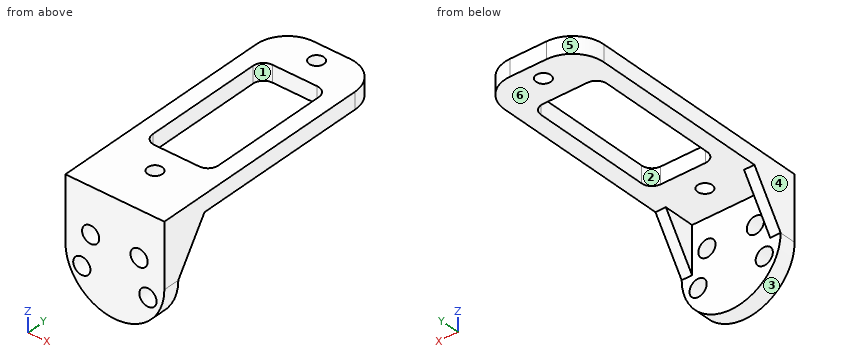
from build123d import *

# Parameters (mm, degrees)
SKETCH1_R               = 1.4
BOSS_EXTRUDE1_DEPTH     = 3.2
BOSS_EXTRUDE3_DEPTH     = 3.2
BOSS_EXTRUDE4_DEPTH     = 2
LPATTERN1_COUNT         = 2
LPATTERN1_PITCH         = 17
CUT_EXTRUDE1_DEPTH      = 54.530365215
CUT_EXTRUDE4_DEPTH      = 54.530365215
CUT_EXTRUDE4_DEPTH_BACK = 54.530365215
SKETCH8_R               = 1.65


with BuildPart() as part:
    # Sketch1 → Boss-Extrude1 (new body)
    with BuildSketch(Plane.XY):
        with BuildLine():
            Line((0, 0), (19, 0))
            Line((19, 0), (19, 40.5))
            ThreePointArc((19, 40.5), (17.242640687, 44.742640687), (13, 46.5))
            Line((13, 46.5), (6, 46.5))
            ThreePointArc((6, 46.5), (1.757359313, 44.742640687), (0, 40.5))
            Line((0, 40.5), (0, 0))
        make_face()
        with Locations((9.5, 6)):
            Circle(SKETCH1_R, mode=Mode.SUBTRACT)
        with Locations((9.5, 43)):
            Circle(SKETCH1_R, mode=Mode.SUBTRACT)
    extrude(amount=BOSS_EXTRUDE1_DEPTH)

    # Sketch2 → Boss-Extrude3 (add)
    with BuildSketch(Plane(origin=(0, 0, 0), x_dir=(1, 0, 0), z_dir=(0, 1, 0))):
        with BuildLine():
            Line((0, 9), (0, -3.2))
            Line((0, -3.2), (19, -3.2))
            Line((19, -3.2), (19, 9))
            ThreePointArc((19, 9), (9.5, 18.5), (0, 9))
        make_face()
    extrude(amount=-BOSS_EXTRUDE3_DEPTH)

    # Sketch3 → Boss-Extrude4 (add)
    with BuildSketch(Plane(origin=(0, 0, 0), x_dir=(0, 0, -1), z_dir=(1, 0, 0))):
        Polygon((0, 0), (9, 0), (0, 6), align=None)
    boss_extrude4 = extrude(amount=BOSS_EXTRUDE4_DEPTH)

    # LPattern1: Boss-Extrude4 ×2
    with Locations(*[(i * LPATTERN1_PITCH, 0, 0) for i in range(1, LPATTERN1_COUNT)]):
        add(boss_extrude4)

    # Sketch4 → Cut-Extrude1 (cut, through all)
    with BuildSketch(Plane.XY):
        with BuildLine():
            Line((5.2, 38), (13.8, 38))
            ThreePointArc((13.8, 38), (15.214213562, 37.414213562), (15.8, 36))
            Line((15.8, 36), (15.8, 13))
            ThreePointArc((15.8, 13), (15.214213562, 11.585786438), (13.8, 11))
            Line((13.8, 11), (5.2, 11))
            ThreePointArc((5.2, 11), (3.785786438, 11.585786438), (3.2, 13))
            Line((3.2, 13), (3.2, 36))
            ThreePointArc((3.2, 36), (3.785786438, 37.414213562), (5.2, 38))
        make_face()
    extrude(amount=CUT_EXTRUDE1_DEPTH, mode=Mode.SUBTRACT)

    # Sketch8 → Cut-Extrude4 (cut, two sides: drawn at the far end of the back side and taken through both)
    with BuildSketch(Plane(origin=(0, 0, 0), x_dir=(1, 0, 0), z_dir=(0, 1, 0)).offset(-CUT_EXTRUDE4_DEPTH_BACK)):
        with Locations(Location((3.15, 11.8, 0), (0, 0, 270))):
            Circle(SKETCH8_R)
        with Locations(Location((14.14852263, 5.45, 0), (0, 0, 270))):
            Circle(SKETCH8_R)
        with Locations(Location((4.85147737, 5.45, 0), (0, 0, 270))):
            Circle(SKETCH8_R)
        with Locations(Location((15.85, 11.8, 0), (0, 0, 270))):
            Circle(SKETCH8_R)
    extrude(amount=CUT_EXTRUDE4_DEPTH + CUT_EXTRUDE4_DEPTH_BACK, mode=Mode.SUBTRACT)


solid = part.part
Source: CAD feature listing. Evaluate the final solid. Frame: model axes, mm. Face numbers are marked on the shaded views. A direction names the side the tool comes from. Round coordinates to 2 decimals unless told otherwise and drop trailing zeros. Loops run counter-clockwise (first coordinate to the right, second up) from the corner with the lowest first, then second, coordinate; pieces in that order, holes last. Notation, with made-up numbers: (38.5, -29.5) -> (64.5, -29.5) arc R17 cw to (64.5, -20.5) -> close; hole circle Ø6 at (10, 20). An arc over 180 degrees is marked (long way). Answer as a JSON object with one key per item and string values. Group by question number.
Q1. Section query A-A (x = 9.5). Output: boundary loops of the cut face in (y, z), plus the area to 3 significant figures.
Q2. Mould query, pull axis X, two halves, no side actions, for the marked faces 1, 2, 3 and 4. Classes: pulls with the +X half, pulls with the -X half, needs draft (parallel to the pull), parting line crosses it, or undercut.
Q3. Contact query for flat-ended pins moving along their axis: P1, Ø6, axis at x = 7.5, z = -11, coming from the +Y side; P2, Ø3, axis at x = 9.5, y = 6, coming from the -Z side. Output: stop coordinate, or through.
Q4. Section query D-D (y = 9). Output: boundary loops of the cut face in (x, z).
Q5. Section query C-C (z = -5.45). Output: boundary loops of the cut face in (x, y), plus the area to 3 significant figures.
Q6. Section query B-B (y = 15). Output: boundary loops of the cut face in (x, z).
Q7. Ray query, line 1 (Y direction, x = 9.5, z = 0.5); line 2 (X direction, y = -2.4, z = -11.8); line 3 (X direction, y = 2, z = -0.25). Return the intervals inside material, ascending. Write a range as from..to.
Q8. Access query for the marked faces 5 and 6. Directions: +Z, -Z, +X, -X, +Y, -Y. A direction counts if a zero-diameter tool reaches every point of the face in a straight line with its end or side. Return the directions, or none.
Completed:
{
 "1": {"outline": "(-3.2, -18.5) -> (0, -18.5) -> (0, 0) -> (4.6, 0) -> (4.6, 3.2) -> (-3.2, 3.2) -> close; (7.4, 0) -> (11, 0) -> (11, 3.2) -> (7.4, 3.2) -> close; (38, 0) -> (41.6, 0) -> (41.6, 3.2) -> (38, 3.2) -> close; (44.4, 0) -> (46.5, 0) -> (46.5, 3.2) -> (44.4, 3.2) -> close", "area": "114 mm²"},
 "2": {"face 1": "undercut", "face 2": "undercut", "face 3": "parting line crosses it", "face 4": "pulls with the -X half"},
 "3": {"P1": "y = 0", "P2": "z = 0"},
 "4": {"outline": "(0, 0) -> (19, 0) -> (19, 3.2) -> (0, 3.2) -> close"},
 "5": {"outline": "(0, -3.2) -> (3.2, -3.2) -> (3.2, 0) -> (2, 0) -> (2, 2.37) -> (0, 2.37) -> close; (6.5, -3.2) -> (12.5, -3.2) -> (12.5, 0) -> (6.5, 0) -> close; (15.8, -3.2) -> (19, -3.2) -> (19, 2.37) -> (17, 2.37) -> (17, 0) -> (15.8, 0) -> close", "area": "49.1 mm²"},
 "6": {"outline": "(0, 0) -> (3.2, 0) -> (3.2, 3.2) -> (0, 3.2) -> close; (15.8, 0) -> (19, 0) -> (19, 3.2) -> (15.8, 3.2) -> close"},
 "7": {"line 1": "-3.2..4.6, 7.4..11, 38..41.6, 44.4..46.5", "line 2": "0.42..1.5, 4.8..14.2, 17.5..18.58", "line 3": "0..2, 17..19"},
 "8": {"face 5": "+Z, -Z, -X, +Y", "face 6": "-Z, +Y"}
}
